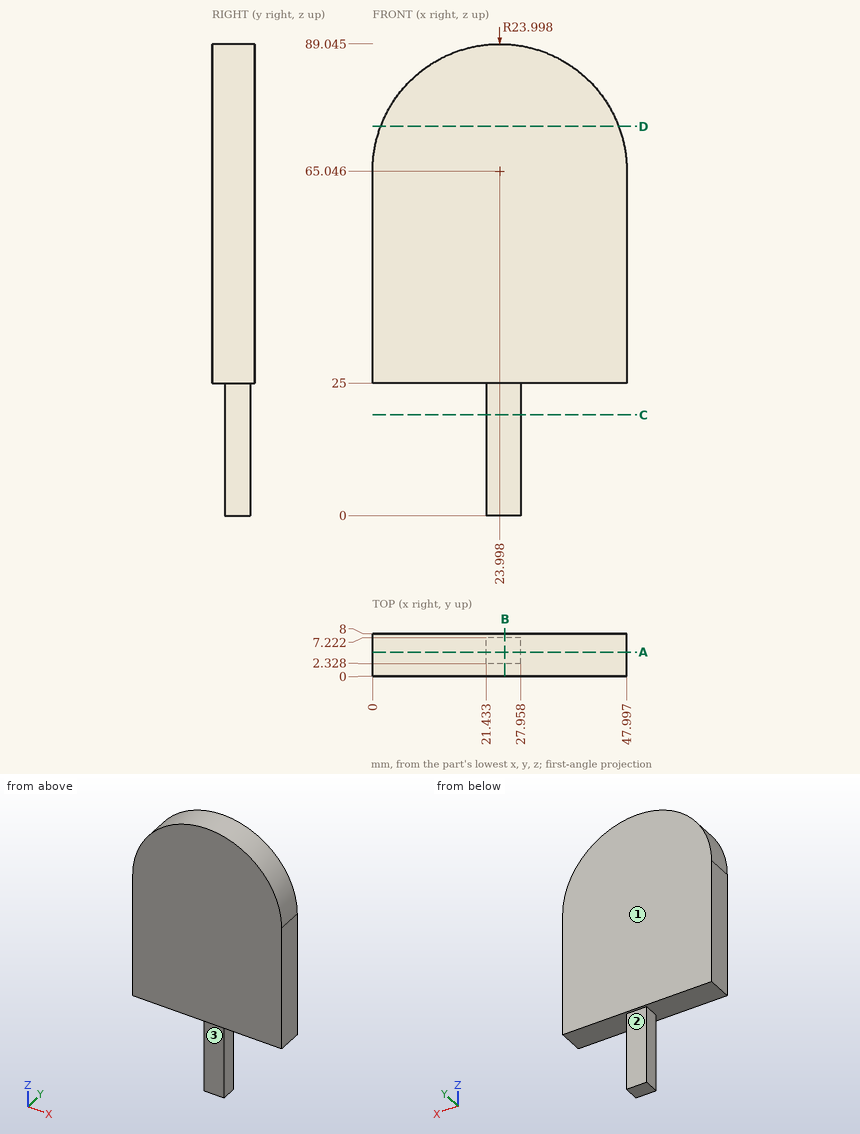
The drawing under review shows one solid part. Ordinate dimensions are in mm from its lowest x, y, z. A direction names the side the tool comes from. Give positions to 0.01 mm unless a question says otherwise; leave off trailing zeros. Write each loop counter-clockwise with the first axis right and the second up, starting at its lowest first coordinate (ties: lowest second). Pieces come first, ordered by that corner, then holes.
1. Tool access review of the marked faces 1, 2 and 3: name each direction out of +Z, -Z, +X, -X, +Y, -Y from which nothing blocks a thin tool from reaching the whole face with its end or side.
2. Add section B-B, the plane x = 25. Write out the cut boundary in (y, z).
3. Add section C-C, the plane z = 19. Write out the cut boundary in (x, y).
4. Wall thickness on L1, parallel to X at y = 5.5, z = 23; L2, parallel to X at y = 7, z = 79 (1 decimal); L3, parallel to Z at x = 17, y = 2.5: over which ranges is each line inside the solid? List them lowest first.
5. Add section A-A, the plane y = 4.5. Write out the cut boundary in (x, z).
6. Add section D-D, the plane z = 73.5. Write out the cut boundary in (x, y), plus the area to 3 significant figures.
7. For P1, Ø2, axis at x = 15, y = 3, coming from the +Z side; P2, Ø10, axis at x = 22.5, z = 44, coming from the -Y side; P3, Ø2.5, axis at x = 14, y = 4, coming from the -Z side; P4, Ø3.5, axis at x = 24, z = 9, coming from the +Y side, all flat-tipped, find the tip position at first contact; note any pin that passes through.
Worked answers:
1. face 1: +Z, -Z, +X, -X, +Y
1. face 2: -Z, +X, -X, +Y
1. face 3: -Z, +X, -X, -Y
2. outline: (0, 25) - (2.33, 25) - (2.33, 0) - (7.22, 0) - (7.22, 25) - (8, 25) - (8, 89.02) - (0, 89.02) - close
3. outline: (21.43, 2.33) - (27.96, 2.33) - (27.96, 7.22) - (21.43, 7.22) - close
4. L1: x = 21.43 to 27.96
4. L2: x = 4.5 to 43.5
4. L3: z = 25 to 88
5. outline: (0, 25) - (21.43, 25) - (21.43, 0) - (27.96, 0) - (27.96, 25) - (48, 25) - (48, 65.05) arc R24 ccw to (0, 65.05) - close
6. outline: (1.54, 0) - (46.46, 0) - (46.46, 8) - (1.54, 8) - close
6. area: 359 mm2
7. P1: stops at z = 87.67
7. P2: stops at y = 0
7. P3: stops at z = 25
7. P4: stops at y = 7.22
